Check sheet for the modelled part. Datum: model origin and axes. Units: mm. Face numbers are marked on the shaded views. A direction names the side the tool comes from. Give positions to 0.01 mm unless a question says otherwise; leave off trailing zeros. Order: outer loops, then holes, each group sorted by start corner. A loop starts at its lowest first (then second) coordinate and runs counter-clockwise, first axis right, second up. Notation, with made-up numbers: (9, -23) - (23, -23) arc R34 ccw to (23, 8) - close; hole circle Ø11 at (-27, 59). An arc over 180 degrees is marked (long way). Answer in a Markdown table with one row per item.
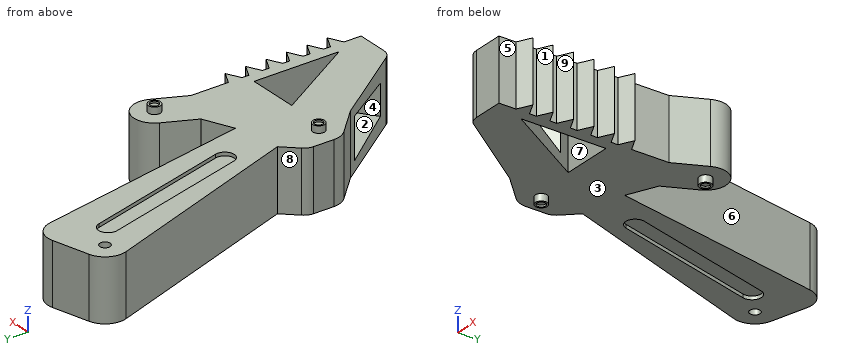
Autodesk Inventor part; units mm, degrees
ref_plane "Work Plane1" through (0, 0, 9) normal (0, 0, 1) x (1, 0, 0)
ref_plane "YZ Plane" through (0, 0, 0) normal (1, 0, 0) x (0, 1, 0)
ref_plane "XZ Plane" through (0, 0, 0) normal (0, 1, 0) x (-1, 0, 0)
sketch "Sketch1" plane through (0, 0, 0) normal (0, 0, 1) x (1, 0, 0)
  line L0 (0, 0) -> (-13.1942, 69.7633)
  line L1 (-13.1942, 69.7633) -> (-36.3853, 63.5848)
  line L2 (-36.3853, 63.5848) -> (-13.3296, -2.5093)
  line L3 (-13.3296, -2.5093) -> (-18.3981, -7.8428)
  line L4 (-18.3981, -7.8428) -> (-18.3981, -17.8428)
  line L5 (-18.3981, -17.8428) -> (-9.2098, -27.0392)
  line L6 (-9.2098, -27.0392) -> (8.4067, -51.3221)
  line L7 (8.4067, -51.3221) -> (19.4067, -51.3221)
  line L8 (19.4067, -51.3221) -> (19.4067, -1.3221)
  line L9 (19.4067, -1.3221) -> (23.6767, 7.7205)
  arc A0 (23.6767, 7.7205) -> (12.8256, 12.8444) centre (18.2512, 10.2824) ccw
  line L10 (8.5557, 3.8018) -> (12.8256, 12.8444)
  line L11 (0, 0) -> (8.5557, 3.8018)
  dimension "d0" = 71
  dimension "d1" = 24
  dimension "d2" = 70
  dimension "d3" = 20
  dimension "d4" = 10
  dimension "d5" = 13
  dimension "d6" = 30
  dimension "d8" = 11
  dimension "d9" = 50
  dimension "d10" = 10
  dimension "d11" = 12
  dimension "d12" = 10
extrude "Extrusion1" add sketch "Sketch1" along normal blind 18
sketch "Sketch2" plane through (0, 0, 18) normal (0, 0, 1) x (1, 0, 0)
  line L0 (16.2045, -42.4982) -> (16.2045, -17.4982)
  line L1 (16.2045, -17.4982) -> (1.2045, -17.4982)
  line L2 (1.2045, -17.4982) -> (16.2045, -42.4982)
  point P0 (0, 0)
  dimension "d15" = 25
  dimension "d16" = 15
extrude "Extrusion2" cut sketch "Sketch2" against normal blind 18
sketch "Sketch3" plane through (0, 0, 18) normal (0, 0, 1) x (1, 0, 0)
  line L0 (19.4067, -51.3221) -> (19.4067, -1.3221) construction
  line L1 (19.4067, -51.3221) -> (19.4067, -46.3221) construction
  line L2 (19.4067, -46.3221) -> (19.4067, -42.3221)
  line L3 (19.4067, -44.3221) -> (23.4067, -44.3221) construction
  line L4 (19.4067, -42.3221) -> (23.4067, -44.3221)
  line L5 (19.4067, -46.3221) -> (23.4067, -44.3221)
  point P0 (0, 0)
  dimension "d19" = 5
  dimension "d20" = 4
  dimension "d21" = 4
extrude "Extrusion3" add sketch "Sketch3" against normal blind 18
pattern_linear "Rectangular Pattern1" count 6 spacing 6 along (0, 1, 0) of "Extrusion3"
fillet "Fillet1" radius 6 3 edges at (-18.3981, -17.8428, 9) (-36.3853, 63.5848, 9) (-13.1942, 69.7633, 9)
fillet "Fillet2" radius 4 2 edges at (-18.3981, -7.8428, 9) (8.4067, -51.3221, 9)
sketch "Sketch5" plane through (0, 0, 18) normal (0, 0, 1) x (1, 0, 0)
  arc A0 (-30.1339, 65.2503) -> (-34.2545, 57.4763) centre (-28.5892, 59.4525) ccw
  circle A1 centre (-28.5892, 59.4525) radius 1.5
  point P0 (0, 0)
  dimension "d32" = 3
extrude "Extrusion5" cut sketch "Sketch5" against normal blind 18
sketch "Sketch6" plane through (-9.2098, -27.0392, 0) normal (-0.8094, -0.5872, 0) x (0, 0, 1)
  line L0 (3, -3) -> (15, -3)
  line L1 (0, 0) -> (0, -27.9601)
  line L2 (18, 0) -> (18, -27.9601)
  line L3 (0, 0) -> (18, 0)
  line L4 (3, -3) -> (4.5418, -23.4291)
  line L5 (18, -23.4291) -> (0, -23.4291)
  line L6 (15, -3) -> (13.4582, -23.4291)
  point P0 (0, 16.4781)
  dimension "d35" = 3
  dimension "d36" = 3
  dimension "d37" = 3
extrude "Extrusion6" cut sketch "Sketch6" against normal blind 14 contours L0 L6 L5 L4
sketch "Sketch7" plane through (0, 0, 18) normal (0, 0, 1) x (1, 0, 0)
  arc A0 (-18.3981, -15.359) -> (-16.6426, -19.5998) centre (-12.3981, -15.359) ccw
  circle A1 centre (-12.3981, -15.359) radius 1.75
  arc A2 (23.6767, 7.7205) -> (12.8256, 12.8444) centre (18.2512, 10.2824) ccw
  circle A3 centre (18.2512, 10.2824) radius 1.75
  point P0 (0, 0)
  dimension "d40" = 3.5
  dimension "d41" = 3.5
extrude "Extrusion7" add sketch "Sketch7" along normal blind 2
sketch "Sketch9" plane through (18.2512, 10.2824, 20) normal (0, 0, 1) x (1, 0, 0)
  circle A0 centre (0, 0) radius 1.75
  circle A1 centre (-30.6493, -25.6415) radius 1.75
  circle A2 centre (0, 0) radius 1.25
  circle A3 centre (-30.6493, -25.6415) radius 1.25
  point P0 (-18.2512, -10.2824)
  dimension "d44" = 0.5
  dimension "d45" = 0.5
extrude "Extrusion8" cut sketch "Sketch9" against normal blind 0.5 contours A2 | A3
sketch "Sketch10" plane through (0, 0, 18) normal (0, 0, 1) x (1, 0, 0)
  line L0 (-21.8945, 53.635) -> (-10.3211, 10.7097) construction
  line L1 (-24.5497, 52.9192) -> (-12.9763, 9.9938)
  line L2 (-7.6659, 11.4256) -> (-19.2393, 54.3509)
  arc A0 (-19.2393, 54.3509) -> (-24.5497, 52.9192) centre (-21.8945, 53.635) ccw
  arc A1 (-12.9763, 9.9938) -> (-7.6659, 11.4256) centre (-10.3211, 10.7097) ccw
  point P0 (0, 0)
  point P1 (-16.1078, 32.1724)
  dimension "d48" = 5.5
extrude "Extrusion9" cut sketch "Sketch10" against normal blind 1
ref_plane "Work Plane1" through (0, 0, 9) normal (0, 0, 1) x (1, 0, 0)
mirror "Mirror1" about plane through (0, 0, 9) normal (0, 0, 1) of "Extrusion9", "Extrusion7", "Extrusion8"
(1) Cross-section at A-A, the plane y = 33.5. Record the cut outline in (x, z).
Geometry says:
| item | result |
|---|---|
| outline | (-25.89, 0) - (-19.31, 0) - (-19.31, 1) - (-13.62, 1) - (-13.62, 0) - (-6.34, 0) - (-6.34, 18) - (-13.62, 18) - (-13.62, 17) - (-19.31, 17) - (-19.31, 18) - (-25.89, 18) - close |
(2) Cross-section at C-C, the plane x = -26. Record the cut outline in (y, z), then the cut area to 3 significant figures.
Geometry says:
| item | result |
|---|---|
| outline | (33.81, 0) - (66.35, 0) - (66.35, 18) - (33.81, 18) - close |
| area | 586 mm² |
(3) Cross-section at B-B, the plane x = -4. Record the cut outline in (y, z), then the cut area to 3 significant figures.
Geometry says:
| item | result |
|---|---|
| outline | (-34.22, 0) - (21.15, 0) - (21.15, 18) - (-34.22, 18) - (-34.22, 14.56) - (-26.97, 15) - (-26.97, 3) - (-34.22, 3.44) - close |
| area | 913 mm² |
(4) Mould release check, pull along Z, two halves, no side actions. Record for the marked faces 1, 2, 3 and 4: pulls with the +Z half, pulls with the -Z half, needs draft (parallel to the pull), parting line crosses it, or undercut.
Geometry says:
| item | result |
|---|---|
| face 1 | needs draft |
| face 2 | undercut |
| face 3 | pulls with the -Z half |
| face 4 | undercut |
(5) Access from +Z, -Z, +X, -X, +Y, -Y to the whole of each face (thin tool, end or side, straight path). Record for the marked faces 5, 6, 7, 8 and 9.
Geometry says:
| item | result |
|---|---|
| face 5 | +Z, -Z, +X, -Y |
| face 6 | +Z, -Z, +Y |
| face 7 | +Z, -Z |
| face 8 | +Z, -Z, -X |
| face 9 | +Z, -Z, +X |
(6) Cross-section at D-D, the plane y = -5.5. Record the cut outline in (x, z), then the cut area to 3 significant figures.
Geometry says:
| item | result |
|---|---|
| outline | (-16.17, 0) - (19.41, 0) - (19.41, 18) - (-16.17, 18) - close |
| area | 640 mm² |
(7) Gauge pin test, flat ends, axial feed: P1, Ø4, axis at y = -49, z = 6.5, coming from the +X side; P2, Ø4, axis at x = -12.4, y = -15.36, coming from the +Z side; P3, Ø10, axis at y = -28.5, z = 15.5, coming from the -X side; P4, Ø1, axis at x = -17.5, z = 16, coming from the -Y side. Record the tip position at first contact, or that the pin passes through.
Geometry says:
| item | result |
|---|---|
| P1 | x = 19.41 |
| P2 | z = 20 |
| P3 | x = -12.75 |
| P4 | y = -19.21 |
(8) Thickness scan on L1, parallel to X at y = -27.5, z = 12.5; L2, parallel to Y at x = 12, z = 7; L3, parallel to X at y = 13, z = 9. Record the ranges inside material, lowest first.
Geometry says:
| item | result |
|---|---|
| L1 | -8.88 to -4.74, 16.2 to 21.05 |
| L2 | -51.32 to -40.6, -17.5 to 11.1 |
| L3 | -18.74 to -2.46, 12.9 to 23.6 |
